Autodesk Inventor part; units mm, degrees
ref_plane "YZ Plane" through (0, 0, 0) normal (1, 0, 0) x (0, 1, 0)
ref_plane "XZ Plane" through (0, 0, 0) normal (0, 1, 0) x (-1, 0, 0)
ref_plane "XY Plane" through (0, 0, 0) normal (0, 0, 1) x (1, 0, 0)
sketch "Sketch1" plane through (0, 0, 0) normal (0, 0, 1) x (1, 0, 0)
  circle A0 centre (0, 0) radius 35
  line L0 (-35, 0) -> (-35, -40)
  line L1 (-35, -40) -> (35, -40)
  line L2 (35, -40) -> (35, 0)
  dimension "d0" = 70
  dimension "d1" = 40
extrude "Extrusion1" add sketch "Sketch1" along normal blind 12.5
sketch "Sketch2" plane through (-35, -40, 0) normal (0, -1, 0) x (1, 0, 0)
  arc A0 (82.5, -22.5) -> (-12.5, -22.5) centre (35, -22.5) ccw
  line L0 (0, 12.5) -> (70, 12.5) construction
  line L1 (35, 12.5) -> (35, 0)
  line L2 (82.5, -22.5) -> (-12.5, -22.5)
  arc A1 (-12.5, -22.5) -> (82.5, -22.5) centre (35, -22.5) ccw construction
  dimension "d4" = 95
  dimension "d6" = 35
extrude "Extrusion2" add sketch "Sketch2" along normal blind 8
chamfer "Chamfer1" distance 3.5 angle 45 3 edges at (0, 35, 12.5) (-35, -20, 12.5) (35, -20, 12.5)
sketch "Sketch3" plane through (0, 0, 0) normal (0, 0, -1) x (-1, 0, 0)
  circle A0 centre (0, 0) radius 12.5
  dimension "d12" = 25
extrude "Extrusion3" cut sketch "Sketch3" against normal blind 5
sketch "Sketch4" plane through (-35, -48, 0) normal (0, -1, 0) x (1, 0, 0)
  arc A0 (82.5, -22.5) -> (-12.5, -22.5) centre (35, -22.5) ccw
  arc A1 (77.5, -22.5) -> (-7.5, -22.5) centre (35, -22.5) ccw
  arc A2 (82.5, -22.5) -> (-12.5, -22.5) centre (35, -22.5) ccw
  line L0 (-7.5, -22.5) -> (-12.5, -22.5)
  line L1 (82.5, -22.5) -> (77.5, -22.5)
  line L2 (-12.5, -22.5) -> (82.5, -22.5)
  circle A3 centre (35, -22.5) radius 32.5
  circle A4 centre (35, -22.5) radius 30
  point P0 (35, 0)
  point P1 (5, -22.5)
  point P2 (65, -22.5)
  point P3 (67.5, -22.5)
  point P4 (2.5, -22.5)
  dimension "d16" = 5
  dimension "d20" = 65
  dimension "d21" = 60
extrude "Extrusion4" cut sketch "Sketch4" against normal blind 4 contours L1 A1 L0 A0 | L2 A4 A3 picked at (43.6934, 7.7339)
properties part number "Base 1 right"
Input: part model. Units: mm. Frame: model coordinates. A direction names the side the tool comes from. Coordinates: 2 decimals unless noted, no trailing zeros. Write each loop counter-clockwise with the first axis right and the second up, starting at its lowest first coordinate (ties: lowest second). Pieces come first, ordered by that corner, then holes. Notation, with made-up numbers: M -6,68 L 10,68 A29 cw 10,95 Z; hole C 52.25,76 d5. An arc over 180 degrees is marked long. Answer as a JSON object with one key per item and string values. Group by question number.
(1) Ray query, line 1 along Y through (x, z) = (0, 2.1); line 2 along Z through (x, y) = (25.5, -15); line 3 along Y through (x, z) = (-40, -16). Return the intervals inside material, ascending. Write a range as [from, to].
(2) Section C-C on y = -17.5. Output: boundary loops of the cut face in (x, z), plus the area to 3 significant figures.
(3) Set-up query: faces 1 (the face through (-35, -20, 4)), 2 (the face through (-4, -44, 21)), 3 (the face through (-11.923, 3.755, 2.465)). Return all of +Z, -Z, +X, -X, +Y, -Y with unobstructed straight access to the full face (end or side cutting, diameter ignored); none if empty.
(4) Section B-B on z = -4. Output: boundary loops of the cut face in (x, y).
(5) Section D-D on z = -9. Output: boundary loops of the cut face in (x, y).
(6) Mould query, pull axis Z, two halves, no side actions, for faces 4 (the face through (0.715, -46.028, 9.992)), 5 (the face through (1, -44, -22.5)), 6 (the face through (3, -48, 11)). Classes: pulls with the +Z half, pulls with the -Z half, needs draft (parallel to the pull), parting line crosses it, or undercut.
(7) Contact query for flat-ended pins moving along their axis: P1, Ø5, axis at x = 23.5, z = -4.5, coming from the +Y side; P2, Ø4.5, axis at y = -13.5, z = 5, coming from the +X side; P3, Ø7, axis at y = -23.5, z = 5.5, coming from the -X side. Output: stop coordinate, or through.
(8) Section A-A on x = 0. Output: boundary loops of the cut face in (y, z).
Result set:
{
 "1": {"line 1": "y = [-48, -12.5], [12.5, 35]", "line 2": "z = [0, 12.5]", "line 3": "y = [-48, -40]"},
 "2": {"outline": "M -35,0 L 35,0 L 35,9 L 31.5,12.5 L -31.5,12.5 L -35,9 Z", "area": "863 mm2"},
 "3": {"face 1": "+Z, -Z, -X, +Y", "face 2": "+Z, -Y", "face 3": "-Z"},
 "4": {"outline": "M -43.75,-44 L -38.26,-44 L -38.26,-48 L -26.72,-48 L -26.72,-44 L -23.62,-44 L -23.62,-48 L 23.62,-48 L 23.62,-44 L 26.72,-44 L 26.72,-48 L 38.26,-48 L 38.26,-44 L 43.75,-44 L 43.75,-40 L -43.75,-40 Z"},
 "5": {"outline": "M -45.54,-44 L -40.3,-44 L -40.3,-48 L -29.56,-48 L -29.56,-44 L -26.79,-44 L -26.79,-48 L 26.79,-48 L 26.79,-44 L 29.56,-44 L 29.56,-48 L 40.3,-48 L 40.3,-44 L 45.54,-44 L 45.54,-40 L -45.54,-40 Z"},
 "6": {"face 4": "undercut", "face 5": "pulls with the -Z half", "face 6": "needs draft"},
 "7": {"P1": "stops at y = -40", "P2": "stops at x = 35", "P3": "stops at x = -35"},
 "8": {"outline": "M -48,-22.5 L -40,-22.5 L -40,0 L -12.5,0 L -12.5,5 L 12.5,5 L 12.5,0 L 35,0 L 35,9 L 31.5,12.5 L -40,12.5 L -40,25 L -44,25 L -44,20 L -48,20 L -48,10 L -44,10 L -44,7.5 L -48,7.5 Z"}
}
